Job drawing, mm, ordinate dimensions from the low corner. One solid piece. A direction names the side the tool comes from. Coordinates: 2 decimals unless noted, no trailing zeros. Write each loop counter-clockwise with the first axis right and the second up, starting at its lowest first coordinate (ties: lowest second). Pieces come first, ordered by that corner, then holes. Notation, with made-up numbers: (32.5, -30) - (49.5, -30) arc R28 ccw to (49.5, -11) - close; hole circle Ø1 at (15, 50.5). An arc over 180 degrees is marked (long way). Use a Markdown table: item, result.
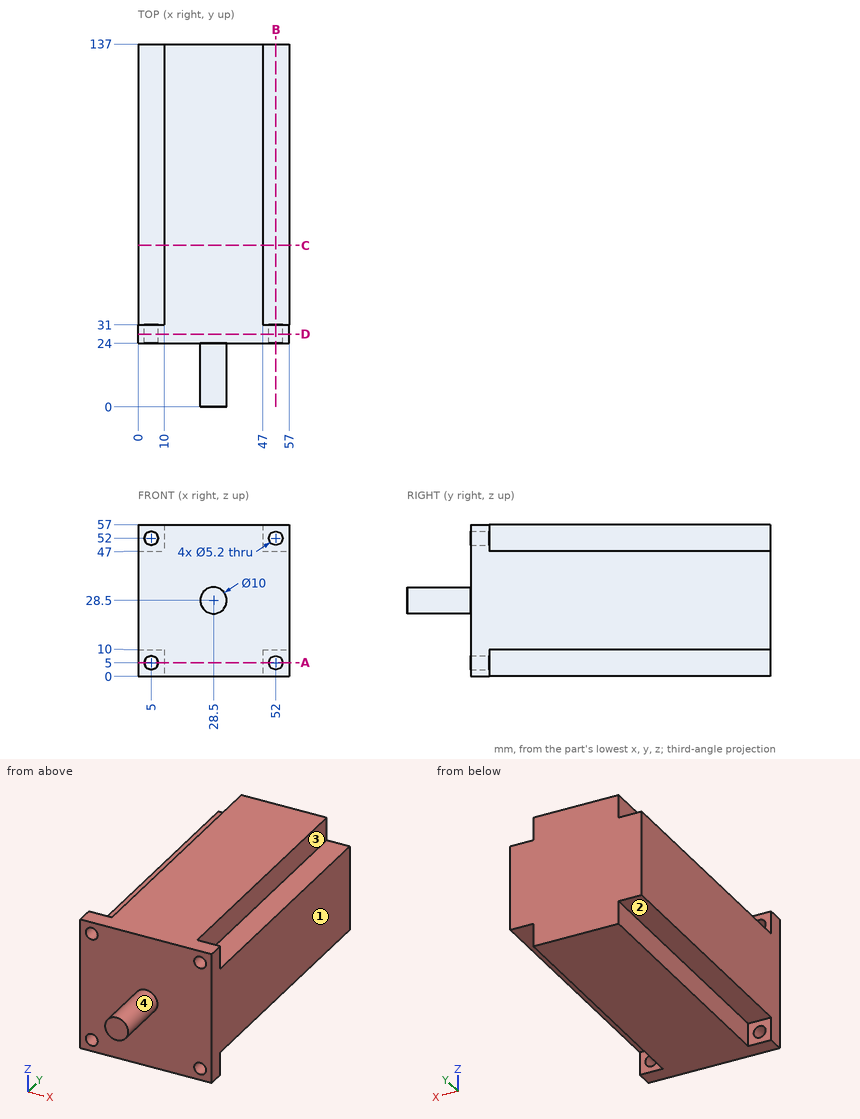
Item 1: Drill centre lines: probe 1 along Z at (x, y) = (5, 28.75); probe 2 along Z at (x, y) = (54, 32.5). Where is each one in solid material? Low to high.
From the geometry:
| item | result |
|---|---|
| probe 1 | 0 to 2.4, 7.6 to 49.4, 54.6 to 57 |
| probe 2 | 10 to 47 |
Item 2: Band-saw the part on A-A, the plane z = 5. Give the cut face in (x, y).
From the geometry:
| item | result |
|---|---|
| outline | (0, 24) - (2.4, 24) - (2.4, 31) - (0, 31) - close; (7.6, 24) - (49.4, 24) - (49.4, 31) - (47, 31) - (47, 137) - (10, 137) - (10, 31) - (7.6, 31) - close; (54.6, 24) - (57, 24) - (57, 31) - (54.6, 31) - close |
Item 3: Band-saw the part on B-B, the plane x = 52. Give the cut face in (y, z), then the cut area to 3 significant figures.
From the geometry:
| item | result |
|---|---|
| outline | (24, 0) - (31, 0) - (31, 2.4) - (24, 2.4) - close; (24, 7.6) - (31, 7.6) - (31, 10) - (137, 10) - (137, 47) - (31, 47) - (31, 49.4) - (24, 49.4) - close; (24, 54.6) - (31, 54.6) - (31, 57) - (24, 57) - close |
| area | 4,250 mm^2 |
Item 4: Which spindle directions (+Z, -Z, +X, -X, +Y, -Y) get a long thin tool onto all of the face, cutting with end or side? Do the marked faces 1, 2, 3 and 4. Say none if no direction does.
From the geometry:
| item | result |
|---|---|
| face 1 | +Z, -Z, +X, +Y, -Y |
| face 2 | -Z, -X, +Y |
| face 3 | +Z, +X, +Y |
| face 4 | -Y |
Item 5: Band-saw the part on D-D, the plane y = 27.5. Give the cut face in (x, z).
From the geometry:
| item | result |
|---|---|
| outline | (0, 0) - (57, 0) - (57, 57) - (0, 57) - close; hole circle Ø5.2 at (5, 5); hole circle Ø5.2 at (5, 52); hole circle Ø5.2 at (52, 5); hole circle Ø5.2 at (52, 52) |
Item 6: Band-saw the part on C-C, the plane y = 61. Give the cut face in (x, z), then the cut area to 3 significant figures.
From the geometry:
| item | result |
|---|---|
| outline | (0, 10) - (10, 10) - (10, 0) - (47, 0) - (47, 10) - (57, 10) - (57, 47) - (47, 47) - (47, 57) - (10, 57) - (10, 47) - (0, 47) - close |
| area | 2,850 mm^2 |
Item 7: Drop flat-ended pins along their axis: P1, Ø8, axis at y = 77.5, z = 52.5, coming from the +X side; P2, Ø3, axis at x = 20, z = 33.5, coming from the -Y side; P3, Ø3, axis at y = 77, z = 50.5, coming from the -X side. Give the stop position or say it passes through.
From the geometry:
| item | result |
|---|---|
| P1 | x = 47 |
| P2 | y = 24 |
| P3 | x = 10 |
